```python
from build123d import *

# Parameters (mm, degrees)
BOSS_EXTRUDE1_DEPTH      = 20
BOSS_EXTRUDE1_DEPTH_BACK = 0.0001
SHELL3_T                 = 3.81
SKETCH9_R                = 1.072598704
BOSS_EXTRUDE3_DEPTH      = 3.001739429
SKETCH19_R               = 1.080792188
BOSS_EXTRUDE4_DEPTH      = 3
BOSS_EXTRUDE5_DEPTH      = 17.32
SKETCH22_W               = 1.806317066
SKETCH22_H               = 1.967276013
SKETCH22_W_2             = 1.806317067
CUT_EXTRUDE1_DEPTH       = 5


with BuildPart() as part:
    # Sketch2 → Boss-Extrude1 (new, two sides: drawn at the far end of the back side and taken through both)
    with BuildSketch(Plane.XY.offset(-BOSS_EXTRUDE1_DEPTH_BACK)):
        Polygon((-6.655720012, 48.566419982), (44.654279988, 48.566419982), (44.654279988, -48.566419982), (-44.654279988, -48.566419982), (-44.654279988, -0.283580018), (-68.655720012, -0.283580018), (-68.655720012, 69.716419982), (-6.655720012, 69.716419982), align=None)
    extrude(amount=BOSS_EXTRUDE1_DEPTH + BOSS_EXTRUDE1_DEPTH_BACK)

    # Shell3
    shell3_openings = [part.faces().sort_by_distance(p)[0] for p in [
        (-10.378060189, 9.486636378, -0.0001),
    ]]
    offset(amount=SHELL3_T, openings=shell3_openings, kind=Kind.INTERSECTION)

    # Sketch9 → Boss-Extrude3 (add)
    with BuildSketch(Plane(origin=(0, 0, 20), x_dir=(-1, 0, 0), z_dir=(0, 0, -1))):
        with BuildLine():
            Line((-44.654279988, 48.566419982), (-38.360252923, 48.566419982))
            ThreePointArc((-38.360252923, 48.566419982), (-40.203730769, 44.115870764), (-44.654279988, 42.272392917))
            Line((-44.654279988, 42.272392917), (-44.654279988, 48.566419982))
        make_face()
        with Locations((-42.441033376, 46.349593762)):
            Circle(SKETCH9_R, mode=Mode.SUBTRACT)
    boss_extrude3 = extrude(amount=BOSS_EXTRUDE3_DEPTH)

    # Mirror1: Boss-Extrude3 across plane
    add(boss_extrude3.mirror(Plane.ZX))

    # Sketch19 → Boss-Extrude4 (add)
    with BuildSketch(Plane(origin=(0, 0, 20), x_dir=(-1, 0, 0), z_dir=(0, 0, -1))):
        with BuildLine():
            Line((39.29950568, -48.566419982), (44.654279988, -48.566419982))
            Line((44.654279988, -48.566419982), (44.654279988, -43.211645674))
            ThreePointArc((44.654279988, -43.211645674), (40.867882763, -44.780022757), (39.29950568, -48.566419982))
        make_face()
        with Locations((42.445754047, -46.356290661)):
            Circle(SKETCH19_R, mode=Mode.SUBTRACT)
    extrude(amount=BOSS_EXTRUDE4_DEPTH)

    # Sketch20 → Boss-Extrude5 (add)
    with BuildSketch(Plane(origin=(0, 0, 20), x_dir=(-1, 0, 0), z_dir=(0, 0, -1))):
        with BuildLine():
            Line((68.655720012, 69.716419982), (68.655720012, 63.716926528))
            ThreePointArc((68.655720012, 63.716926528), (64.413437506, 65.474137477), (62.656226557, 69.716419982))
            Line((62.656226557, 69.716419982), (68.655720012, 69.716419982))
        make_face()
        with BuildLine():
            Line((68.655720012, 5.716419982), (68.655720012, -0.283580018))
            Line((68.655720012, -0.283580018), (62.655720012, -0.283580018))
            ThreePointArc((62.655720012, -0.283580018), (64.413079325, 3.959060669), (68.655720012, 5.716419982))
        make_face()
    extrude(amount=BOSS_EXTRUDE5_DEPTH)

    # Sketch22 → Cut-Extrude1 (cut)
    with BuildSketch(Plane(origin=(0, 0, -0.0001), x_dir=(-1, 0, 0), z_dir=(0, 0, -1))):
        with Locations((46.539737407, -50.361848815)):
            Rectangle(SKETCH22_W, SKETCH22_H)
        with Locations((46.696837753, -2.332274853)):
            Rectangle(SKETCH22_W, SKETCH22_H)
        with Locations((-46.38572761, -50.279884702)):
            Rectangle(SKETCH22_W_2, SKETCH22_H)
        with Locations((-46.582637328, 50.219582477)):
            Rectangle(SKETCH22_W_2, SKETCH22_H)
        with Locations((4.657343006, 50.463554198)):
            Rectangle(SKETCH22_W_2, SKETCH22_H)
    extrude(amount=-CUT_EXTRUDE1_DEPTH, mode=Mode.SUBTRACT)


solid = part.part
```
Design review of the part built by this model. Coordinates are the model's own, in mm. A direction names the side the tool comes from. Round coordinates to 2 decimals unless told otherwise and drop trailing zeros. Write each loop counter-clockwise with the first axis right and the second up, starting at its lowest first coordinate (ties: lowest second). Pieces come first, ordered by that corner, then holes. Notation, with made-up numbers: (-35.5, -38.75) -> (-28.5, -38.75) arc R27 cw to (-28.5, -0.75) -> close; hole circle Ø7 at (-3, 35). An arc over 180 degrees is marked (long way). Answer in a Markdown table with one row per item.
Q1. Take a section at A-A, the plane z = 15.25. State the section outline as (x, y) points.
The answers:
| item | result |
|---|---|
| outline | (-72.47, -4.09) -> (-48.46, -4.09) -> (-48.46, -52.38) -> (48.46, -52.38) -> (48.46, 52.38) -> (-2.85, 52.38) -> (-2.85, 73.53) -> (-72.47, 73.53) -> close; hole (-68.66, 5.72) arc R6 cw to (-62.66, -0.28) -> (-44.65, -0.28) -> (-44.65, -48.57) -> (44.65, -48.57) -> (44.65, 48.57) -> (-6.66, 48.57) -> (-6.66, 69.72) -> (-62.66, 69.72) arc R6 cw to (-68.66, 63.72) -> close |
Q2. Take a section at C-C, the plane y = -29.5. State the section outline as (x, z) points, then the cut area to 3 significant figures.
The answers:
| item | result |
|---|---|
| outline | (-48.46, 0) -> (-44.65, 0) -> (-44.65, 20) -> (44.65, 20) -> (44.65, 0) -> (48.46, 0) -> (48.46, 23.81) -> (-48.46, 23.81) -> close |
| area | 522 mm² |
Q3. Draft analysis for pull direction X (two halves, no side actions). For faces 1 (the face through (44.654, 1, 10)), 2 (the face through (-72.466, 34, 12)), 3 (the face through (-11, 11, 23.81)), 4 (the face through (48.464, 1, 12)), state which applies: +X half, -X half, draft (parallel to the pull), parting line (faces both ways), or undercut.
The answers:
| item | result |
|---|---|
| face 1 | undercut |
| face 2 | -X half |
| face 3 | draft |
| face 4 | +X half |
Q4. To check wall thickness, follow L1, parallel to Y at x = 41, z = 8; L2, parallel to X at y = -24.5, z = 18; L3, parallel to Y at x = -54, z = 16. State the ranges of each line that lie inside material, in increasing order. Write a range as [from, to].
The answers:
| item | result |
|---|---|
| L1 | [-52.38, -48.57], [48.57, 52.38] |
| L2 | [-48.46, -44.65], [44.65, 48.46] |
| L3 | [-4.09, -0.28], [69.72, 73.53] |
Q5. Clearance check with flat-ended pins moving along their axes: pin 1 Ø0.5 at (x, z) = (46, 1.5) entering from +Y; pin 2 Ø6 at (x, y) = (-43, -46) entering from -Z; pin 3 Ø1.9 at (x, y) = (43, 44) entering from -Z; pin 4 Ø12 at (y, z) = (-32.5, 16) entering from -X. State where each tip first meets the part, or that it passes through.
The answers:
| item | result |
|---|---|
| pin 1 | y = 52.38 |
| pin 2 | z = 0 |
| pin 3 | z = 17 |
| pin 4 | x = -48.46 |
Q6. Take a section at B-B, the plane x = 29.5. State the section outline as (y, z) points.
The answers:
| item | result |
|---|---|
| outline | (-52.38, 0) -> (-48.57, 0) -> (-48.57, 20) -> (48.57, 20) -> (48.57, 0) -> (52.38, 0) -> (52.38, 23.81) -> (-52.38, 23.81) -> close |
Q7. For faces 5 (the face through (1, -48.566, 10)), 6 (the face through (-2.846, 63, 12)), 7 (the face through (-48.464, -29, 12)), list the 3-axis set-ups (+Z, -Z, +X, -X, +Y, -Y) from which the entire face can be reached by the end or side of a thin tool; tool diameter is ignored.
The answers:
| item | result |
|---|---|
| face 5 | -Z |
| face 6 | +Z, -Z, +X, +Y |
| face 7 | +Z, -Z, -X, -Y |
